Input: part model. Units: mm. Frame: model coordinates. A direction names the side the tool comes from. Give positions to 0.01 mm unless a question says otherwise; leave off trailing zeros. Order: outer loops, then holes, each group sorted by start corner. A loop starts at its lowest first (then second) coordinate and runs counter-clockwise, first axis right, second up. Notation, with made-up numbers: (60.25, -1) - (94.25, -1) arc R6 ccw to (94.25, 6) - close; hole circle Ø1 at (-20.75, 89.25). An arc over 180 degrees is marked (long way). Answer in a Markdown table with one row per item. Add a question column.
Autodesk Inventor part; units mm, degrees
ref_plane "YZ Plane" through (0, 0, 0) normal (1, 0, 0) x (0, 1, 0)
ref_plane "XZ Plane" through (0, 0, 0) normal (0, 1, 0) x (-1, 0, 0)
ref_plane "XY Plane" through (0, 0, 0) normal (0, 0, 1) x (1, 0, 0)
sketch "Sketch1" plane through (0, 0, 0) normal (0, 0, 1) x (1, 0, 0)
  line L0 (14.2875, 0) -> (14.2875, 5.08)
  line L1 (14.2875, 5.08) -> (15.875, 5.08)
  line L2 (12.7, 7.62) -> (12.7, 0)
  line L3 (12.7, 0) -> (14.2875, 0)
  line L4 (0, -2.54) -> (0, 15.24)
  line L5 (14.2875, 12.7) -> (14.2875, 7.62)
  line L6 (14.2875, 7.62) -> (15.875, 7.62)
  line L7 (15.875, 7.62) -> (15.875, 5.08)
  line L8 (15.875, 7.62) -> (15.875, 12.7)
  line L9 (15.875, 12.7) -> (14.2875, 12.7)
  line L10 (12.7, 7.62) -> (14.2875, 7.62)
  point P0 (0, 0)
  dimension "d1" = 14.2875
  dimension "d2" = 12.7
  dimension "d3" = 5.08
revolve "Revolution1" add sketch "Sketch1" angle 360 about axis through (0, -10, 0) along (0, 1, 0) contours L3 L2 L10 L6 L7 L1 L0
thread "Thread4"
sketch "Sketch5" plane through (0, 0, 0) normal (1, 0, 0) x (0, 1, 0)
  line L0 (-0.3529, -13.8698) -> (-0.3025, -13.8698) construction
  line L1 (0.0503, -14.2571) -> (-0.0001, -14.3539) construction
  line L2 (-0.6049, -14.3539) -> (-0.6553, -14.2571) construction
  line L3 (-0.2521, -13.8698) -> (-0.3025, -13.773) construction
  line L4 (-0.3025, -13.773) -> (-0.3529, -13.8698) construction
  line L5 (-0.6049, -14.3539) -> (-0.5545, -14.2571) construction
  line L6 (-0.2521, -13.8698) -> (-0.0505, -14.2571)
  line L7 (-0.6553, -14.2571) -> (-0.5545, -14.2571) construction
  arc A0 (-0.6553, -14.2571) -> (-0.6049, -14.2877) centre (-0.6049, -14.2309) ccw construction
  line L8 (0.0503, -14.2571) -> (-0.0505, -14.2571) construction
  line L9 (-0.6049, -14.3539) -> (-0.6049, -14.2571) construction
  line L10 (-0.0001, -14.3539) -> (-0.0001, -14.2571) construction
  line L11 (-0.3025, -13.773) -> (-0.3025, -13.8393) construction
  line L12 (-0.6049, -14.2877) -> (-0.0001, -14.2877)
  arc A1 (-0.6049, -14.2877) -> (-0.5545, -14.2571) centre (-0.6049, -14.2309) ccw
  line L13 (-0.0505, -14.2571) -> (-0.0001, -14.3539) construction
  line L14 (-0.5545, -14.2571) -> (-0.3529, -13.8698)
  line L15 (-0.0001, -0.0002) -> (-0.0001, 0.0177)
  line L16 (-0.0001, 0.0177) -> (-0.0001, -0.0002)
  line L17 (-0.0001, -0.0002) -> (0.0334, -0.0002)
  arc A2 (-0.0505, -14.2571) -> (-0.0001, -14.2877) centre (-0.0001, -14.2309) ccw
  arc A3 (-0.0001, -14.2877) -> (0.0503, -14.2571) centre (-0.0001, -14.2309) ccw construction
  arc A4 (-0.3025, -13.8393) -> (-0.3529, -13.8698) centre (-0.3025, -13.8961) ccw
  arc A5 (-0.2521, -13.8698) -> (-0.3025, -13.8393) centre (-0.3025, -13.8961) ccw
  line L18 (-0.3025, -13.8393) -> (-0.3025, -13.8698) construction
  line L19 (-0.3025, -13.8698) -> (-0.2521, -13.8698) construction
  dimension "d31" = 55
  dimension "d32" = 0.0968
  dimension "d33" = 0.0968
  dimension "Sketch5_ThreadOffset" = 0
  dimension "Sketch5_MajorRadius" = 14.2875
  dimension "d36" = 0.6048
  dimension "Sketch5_MinorRadius" = 13.8391
sketch "Sketch6" plane through (0, 0, 0) normal (-1, 0, 0) x (0, 0, 1)
  line L0 (14.2875, 0) -> (14.2875, 5.08)
  line L1 (14.2875, 5.08) -> (13.8391, 5.08)
  line L2 (13.8391, 5.08) -> (13.8391, 0)
  line L3 (13.8391, 0) -> (14.2875, 0)
  line L4 (0, -1.016) -> (0, 6.096)
sketch "Sketch7" plane through (0, 0, 0) normal (-1, 0, 0) x (0, 0, 1)
  line L0 (14.2875, 0) -> (14.2875, 5.08)
  line L1 (14.2875, 5.08) -> (13.8391, 5.08)
  line L2 (13.8391, 5.08) -> (13.8391, 0)
  line L3 (13.8391, 0) -> (14.2875, 0)
  line L4 (0, -1.016) -> (0, 6.096)
equation "\"d31\" = d38"
equation "\"d32\" = 0.160083 * Sketch5_Pitch"
equation "\"d33\" = 0.160083 * Sketch5_Pitch"
equation "\"d36\" = Sketch5_Pitch"
equation "\"d15\" = 55deg"
equation "\"Sketch2_Pitch\" = 0.90714"
equation "\"d38\" = 55deg"
equation "\"Sketch5_Pitch\" = 0.60476"
properties part number "202-experiment"
Q1. Access query for faces 4 (the cylindrical face through (-3.441, 6.332, -15.497)), 5 (the flat face through (-11.83, 5.08, -8.31)). Directions: +Z, -Z, +X, -X, +Y, -Y. A direction counts if a zero-diameter tool reaches every point of the face in a straight line with its end or side. Return the directions, or none.
Q2. Pull-direction query (X, two-part tool) for faces 1 (the cylindrical face through (-2.75, 3.76, -12.4)), 2 (the cylindrical face through (-14.274, 2.576, -0.628)), 3 (the flat face through (-7, 7.62, -11)); classes: +X half, -X half, draft (parallel to the pull), parting line (faces both ways), or undercut.
Q3. Line query: probe 1 along X at (y, z) = (2, 0); probe 2 along Z at (x, y) = (0, 6.25) (3 decimals). Output: solid intervals per line, ascending.
Q4. Section C-C, the plane y = 2.25. Return loops of the section in (x, z) (1 decimal), then the cut area to 3 significant figures.
Q5. Section A-A, the plane x = 0. Return loops of the section in (y, z) (1 decimal).
Q6. Section B-B, the plane z = 0. Return loops of the section in (x, y) (1 decimal).
Q7. Contact query for flat-ended pins moving along their axis: P1, Ø1.5, axis at y = 1.5, z = -8, coming from the +X side; P2, Ø2, axis at x = 11.5, y = 2, coming from the +Z side; P3, Ø2, axis at y = 1.5, z = 12.5, coming from the +X side. Output: stop coordinate, or through.
Computed:
| question | item | result |
|---|---|---|
| 1 | face 4 | +Y, -Y |
| 1 | face 5 | -Y |
| 2 | face 1 | undercut |
| 2 | face 2 | parting line |
| 2 | face 3 | draft |
| 3 | probe 1 | x = -14.29 to -12.7, 12.7 to 14.29 |
| 3 | probe 2 | z = -15.875 to -12.7, 12.7 to 15.875 |
| 4 | outline | circle Ø28.6 at (0, 0); hole circle Ø25.4 at (0, 0) |
| 4 | area | 135 mm^2 |
| 5 | outline | (0, -14.3) - (5.1, -14.3) - (5.1, -15.9) - (7.6, -15.9) - (7.6, -12.7) - (0, -12.7) - close; (0, 12.7) - (7.6, 12.7) - (7.6, 15.9) - (5.1, 15.9) - (5.1, 14.3) - (0, 14.3) - close |
| 6 | outline | (-15.9, 5.1) - (-14.3, 5.1) - (-14.3, 0) - (-12.7, 0) - (-12.7, 7.6) - (-15.9, 7.6) - close; (12.7, 0) - (14.3, 0) - (14.3, 5.1) - (15.9, 5.1) - (15.9, 7.6) - (12.7, 7.6) - close |
| 7 | P1 | stops at x = 12.31 |
| 7 | P2 | stops at z = 9.69 |
| 7 | P3 | stops at x = 8.48 |
